Design review of the part built by this model. Coordinates are the model's own, in mm. Round coordinates to 2 decimals unless told otherwise and drop trailing zeros. Order: outer loops, then holes, each group sorted by start corner. A loop starts at its lowest first (then second) coordinate and runs counter-clockwise, first axis right, second up.
from build123d import *

# Parameters (mm, degrees)
F1_DEPTH = 20


with BuildPart() as f1:
    # F0 (on Right) → F1 (new body)
    with BuildSketch(Plane.YZ):
        Polygon((-132.7905619136, 20), (-132.7905619136, 0), (-104.3375672974, 0), (-104.3375672974, 20), (-4.3375672974, 20), (-4.3375672974, 0), (15.6624327026, 0), (27.2094380864, 20), (160, 250), (0, 250), align=None)
        Polygon((27.2094380864, 20), (15.6624327026, 0), (27.2094380864, 0), align=None)
        Polygon((0, 350), (0, 250), (160, 250), (160, 350), (140, 350), (140, 330), (40, 330), (40, 350), align=None)
    extrude(amount=F1_DEPTH)


solid = f1.part
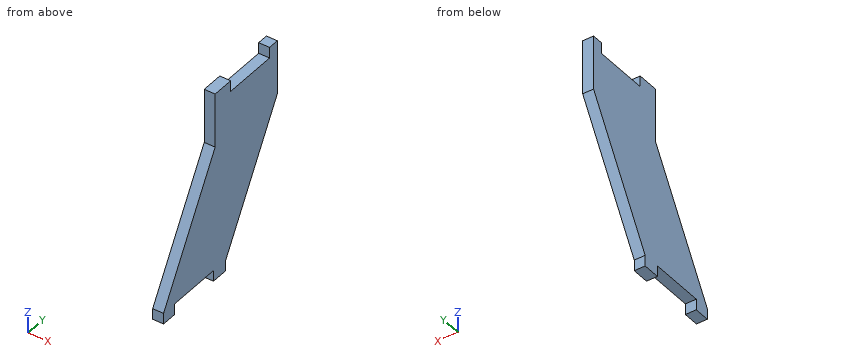
1) To check wall thickness, follow line 1 along Y through (x, z) = (16.75, 273.5); line 2 along Z through (x, y) = (9.75, -8); line 3 along Z through (x, y) = (4, 28). State the ranges of each line that lie inside material, in increasing order.
Results:
line 1: y = 0 to 160
line 2: z = 20 to 236.14
line 3: z = 21.37 to 350
2) Take a section at C-C on y = -58. Give the boundary of the cut face in (x, z), plus the area to 3 significant figures.
Results:
outline: (0, 20) - (20, 20) - (20, 149.54) - (0, 149.54) - close
area: 2,590 mm2
3) Take a section at B-B on z = 276. Give the boundary of the cut face in (x, y).
Results:
outline: (0, 0) - (20, 0) - (20, 160) - (0, 160) - close
4) Clearance check with flat-ended pins moving along their axes: P1, Ø8, axis at x = 6.5, z = 258.5, coming from the -Y side; P2, Ø8, axis at x = 8, z = 232, coming from the -Y side; P3, Ø5, axis at x = 9.5, z = 171.5, coming from the +Y side. State where each tip first meets the part, or that it passes through.
Results:
P1: stops at y = 0
P2: stops at y = -12.7
P3: stops at y = 116.12
5) Take a section at A-A on x = 13. Give the boundary of the cut face in (y, z).
Results:
outline: (-132.79, 0) - (-104.34, 0) - (-104.34, 20) - (-4.34, 20) - (-4.34, 0) - (27.21, 0) - (27.21, 20) - (160, 250) - (160, 350) - (140, 350) - (140, 330) - (40, 330) - (40, 350) - (0, 350) - (0, 250) - (-132.79, 20) - close
